from build123d import *

# Parameters (mm, degrees)
F1_DEPTH   = 50
F1_FACE1_W = 25
F1_FACE1_H = 100
F3_DEPTH   = 6
F5_DEPTH   = 25
F6_W       = 25
F6_H       = 8
F7_DEPTH   = 3
F9_D       = 3.3


with BuildPart() as f1:
    # F0 (on Front) → F1 (new body, symmetric)
    with BuildSketch(Plane.XZ):
        Polygon((-16.8301270189, 2), (-14.5, 2), (-14.5, 0), (14.5, 0), (14.5, 2), (16.8301270189, 2), (12.5, 9.5), (-12.5, 9.5), align=None)
    extrude(amount=F1_DEPTH, both=True)

    # F2 (on face) + F1_face1 (on face) → F3 (cut)
    with BuildSketch(Plane(origin=(0, 0, 0), x_dir=(1, 0, 0), z_dir=(0, 0, -1))):
        with BuildLine():
            Line((4.5, -42), (4.5, -7))
            ThreePointArc((4.5, -7), (0, -2.5), (-4.5, -7))
            Line((-4.5, -7), (-4.5, -42))
            Line((-4.5, -42), (-4.5, -42.0004010455))
            ThreePointArc((-4.4999999821, -42.0004010455), (0.0002005227, -46.4999999955), (4.5, -42))
        make_face()
    with BuildSketch(Plane.XY.offset(9.5)):
        Rectangle(F1_FACE1_W, F1_FACE1_H)
    extrude(amount=-F3_DEPTH, dir=(0, 0, -1), mode=Mode.SUBTRACT)

    # F4 (on face) → F5 (cut)
    with BuildSketch(Plane.XY.offset(9.5)):
        with BuildLine():
            ThreePointArc((-1.9907275363, 7.1923639157), (-0.0962936325, 5.0023194609), (2, 7))
            ThreePointArc((2, 7), (0.0962936325, 8.9976805391), (-1.9907275363, 7.1923639157))
        make_face()
        with BuildLine():
            Line((2, 7), (2, 42))
            ThreePointArc((2, 42), (0.0002663937, 40.0000000177), (-1.999999929, 41.9994672126))
            Line((-1.999999929, 41.9994672126), (-1.9907275363, 7.1923639157))
            ThreePointArc((-1.9907275363, 7.1923639157), (0.0962936325, 8.9976805391), (2, 7))
        make_face()
        with BuildLine():
            ThreePointArc((-1.999999929, 41.9994672126), (0.0002663937, 40.0000000177), (2, 42))
            ThreePointArc((2, 42), (-0.0002663937, 43.9999999823), (-1.999999929, 41.9994672126))
        make_face()
    extrude(amount=-F5_DEPTH, mode=Mode.SUBTRACT)

    # F6 (on face) → F7 (cut)
    with BuildSketch(Plane.XY.offset(9.5)):
        with Locations((0, -46)):
            Rectangle(F6_W, F6_H)
        Polygon((-23.7841614955, -55.5199324694), (24.0457867705, -55.5199324694), (24.0457867705, -42), (12.5, -42), (12.5, -50), (-12.5, -50), (-12.5, -42), (-23.7841614955, -42), align=None)
    extrude(amount=-F7_DEPTH, mode=Mode.SUBTRACT)

    # F9 (through all)
    with Locations(Plane.XY.offset(6.5)):
        with Locations((-7.5, -46), (7.5, -46)):
            Hole(F9_D / 2)


solid = f1.part
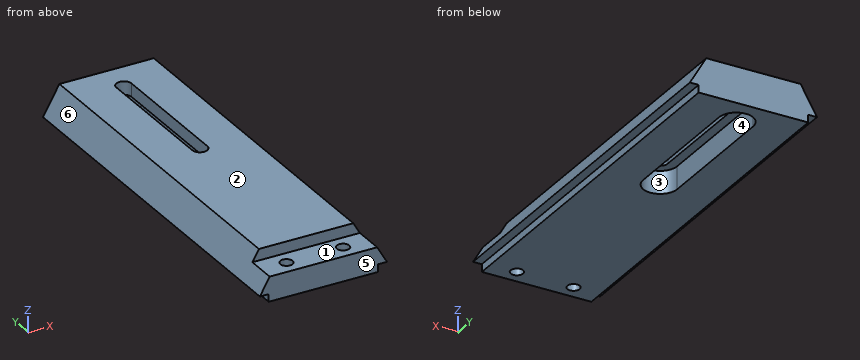
Could you check a few things on this model? Use its own coordinates, in mm. Face numbers are marked on the shaded views. A direction names the side the tool comes from. Give positions to 0.01 mm unless a question says otherwise; leave off trailing zeros. Loops run counter-clockwise (first coordinate to the right, second up) from the corner with the lowest first, then second, coordinate; pieces in that order, holes last. Notation, with made-up numbers: (-27.5, 11) -> (8.5, 11) arc R21 ccw to (8.5, 36) -> close; hole circle Ø4 at (-34, -14). An arc over 180 degrees is marked (long way). Return JSON: item names as keys, results as strings.
Item 1: If we section it at A-A on y = -46: List the corners of the cut face in (x, z) for me, plus the area to 3 significant figures.
Geometry results:
{"outline": "(-16.83, 2) -> (-14.5, 2) -> (-14.5, 0) -> (-9.15, 0) -> (-9.15, 6.5) -> (-14.23, 6.5) -> close; (-5.85, 0) -> (5.85, 0) -> (5.85, 6.5) -> (-5.85, 6.5) -> close; (9.15, 0) -> (14.5, 0) -> (14.5, 2) -> (16.83, 2) -> (14.23, 6.5) -> (9.15, 6.5) -> close", "area": "155 mm²"}
Item 2: I need wall thicknesses on L1, parallel to Y at x = -7.5, z = 3.5; L2, parallel to X at y = 18, z = 1.5; L3, parallel to Y at x = 1, z = 5.75. Which ranges of each line are inside material? Lowest first, please. Write a range as from..to.
Geometry results:
{"L1": "y = -50..-47.65, -44.35..50", "L2": "x = -14.5..-4.5, 4.5..14.5", "L3": "y = -50..2.61, 46.39..50"}
Item 3: We'd pull the mould along Y, two halves only. Please class the marked faces 4, 5 and 6: +Y half, -Y half, draft (parallel to the pull), parting line (faces both ways), or undercut.
Geometry results:
{"face 4": "undercut", "face 5": "-Y half", "face 6": "draft"}
Item 4: Which directions (+Z, -Z, +X, -X, +Y, -Y) give clear straight access to the entire face, cutting with the end or side of a thin tool? Please do the marked faces 1, 2 and 3.
Geometry results:
{"face 1": "+Z, +X, -X, -Y", "face 2": "+Z, +X, -X, +Y, -Y", "face 3": "-Z"}
Item 5: If we section it at D-D on y = 18.5: List the corners of the cut face in (x, z) for me.
Geometry results:
{"outline": "(-16.83, 2) -> (-14.5, 2) -> (-14.5, 0) -> (-4.5, 0) -> (-4.5, 6) -> (-1.99, 6) -> (-1.99, 9.5) -> (-12.5, 9.5) -> close; (2, 6) -> (4.5, 6) -> (4.5, 0) -> (14.5, 0) -> (14.5, 2) -> (16.83, 2) -> (12.5, 9.5) -> (2, 9.5) -> close"}
Item 6: If we section it at B-B on x = 7.5: List the corners of the cut face in (y, z) for me.
Geometry results:
{"outline": "(-50, 0) -> (-47.65, 0) -> (-47.65, 6.5) -> (-50, 6.5) -> close; (-44.35, 0) -> (50, 0) -> (50, 9.5) -> (-42, 9.5) -> (-42, 6.5) -> (-44.35, 6.5) -> close"}
Item 7: I'm going to push flat-ended pins straight in: pin 1 (0.6 mm diameter, centred on y = -19.5, z = 0.5, fed in from +X); pin 2 (1.8 mm diameter, centred on y = 25.5, z = 7.5, fed in from +X); pin 3 (1 mm diameter, centred on y = 35, z = 8, fed in from -X). Where does each tip first touch, or does it pass through?
Geometry results:
{"pin 1": "stops at x = 14.5", "pin 2": "stops at x = 14.17", "pin 3": "stops at x = -13.65"}
Item 8: If we section it at C-C on z = 1: List the corners of the cut face in (x, y) for me, plus the area to 3 significant figures.
Geometry results:
{"outline": "(-14.5, -50) -> (14.5, -50) -> (14.5, 50) -> (-14.5, 50) -> close; hole circle Ø3.3 at (-7.5, -46); hole (-4.5, 7) arc R4.5 ccw to (4.5, 7) -> (4.5, 42) arc R4.5 ccw to (-4.5, 42) -> close; hole circle Ø3.3 at (7.5, -46)", "area": "2,500 mm²"}
